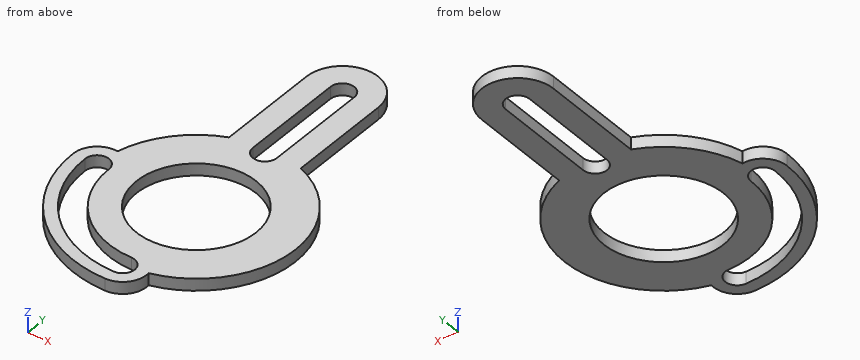
from build123d import *

# Parameters (mm, degrees)
SKETCH2_R           = 25
BOSS_EXTRUDE1_DEPTH = 5


with BuildPart() as part:
    # Sketch2 → Boss-Extrude1 (new body)
    with BuildSketch(Plane.XY):
        with BuildLine():
            Line((15, 82.39), (15, 38.694314828))
            ThreePointArc((15, 38.694314828), (41.414681799, -2.659723947), (9.927155207, -40.295180723))
            ThreePointArc((9.927155207, -40.295180723), (7.484924608, -48.131432999), (0, -51.5))
            ThreePointArc((0, -51.5), (-36.415999231, -36.415999231), (-51.5, 0))
            ThreePointArc((-51.5, 0), (-48.131432999, 7.484924608), (-40.295180723, 9.927155207))
            ThreePointArc((-40.295180723, 9.927155207), (-31.16531118, 27.403893502), (-15, 38.694314828))
            Line((-15, 38.694314828), (-15, 82.39))
            ThreePointArc((-15, 82.39), (0, 97.39), (15, 82.39))
        make_face()
        Circle(SKETCH2_R, mode=Mode.SUBTRACT)
        with BuildLine():
            Line((-5, 38.69), (-5, 82.39))
            ThreePointArc((-5, 82.39), (0, 87.39), (5, 82.39))
            Line((5, 82.39), (5, 38.69))
            ThreePointArc((5, 38.69), (0, 33.69), (-5, 38.69))
        make_face(mode=Mode.SUBTRACT)
        with BuildLine():
            ThreePointArc((-46.5, 0), (-32.880465325, -32.880465325), (0, -46.5))
            ThreePointArc((0, -46.5), (5, -41.5), (0, -36.5))
            ThreePointArc((0, -36.5), (-25.809397513, -25.809397513), (-36.5, 0))
            ThreePointArc((-36.5, 0), (-41.5, 5), (-46.5, 0))
        make_face(mode=Mode.SUBTRACT)
    extrude(amount=BOSS_EXTRUDE1_DEPTH)


solid = part.part
For this review, take the finished solid that the model builds, in its own axes (mm). Round coordinates to 2 decimals unless told otherwise and drop trailing zeros. Loops run counter-clockwise (first coordinate to the right, second up) from the corner with the lowest first, then second, coordinate; pieces in that order, holes last. Notation, with made-up numbers: (38, 26.5) - (69, 26.5) arc R27 ccw to (69, 56.5) - close; hole circle Ø4 at (23, -9). An arc over 180 degrees is marked (long way). Use one line per item in the form item = value.
Item 1: Consider section A-A on z = 0.95. Write out the cut boundary in (x, y).
Answers:
outline = (-51.5, 0) arc R51.5 ccw to (0, -51.5) arc R10 ccw to (9.93, -40.3) arc R41.5 ccw to (15, 38.69) - (15, 82.39) arc R15 ccw to (-15, 82.39) - (-15, 38.69) arc R41.5 ccw to (-40.3, 9.93) arc R10 ccw to start; hole (-46.5, 0) arc R46.5 ccw to (0, -46.5) arc R5 ccw to (0, -36.5) arc R36.5 cw to (-36.5, 0) arc R5 ccw to start; hole circle Ø50 at (0, 0); hole (-5, 38.69) arc R5 ccw to (5, 38.69) - (5, 82.39) arc R5 ccw to (-5, 82.39) - close
Item 2: Consider section D-D on x = -3. Write out the cut boundary in (y, z).
Answers:
outline = (-51.41, 0) - (-46.4, 0) - (-46.4, 5) - (-51.41, 5) - close; (-36.38, 0) - (-24.82, 0) - (-24.82, 5) - (-36.38, 5) - close; (24.82, 0) - (34.69, 0) - (34.69, 5) - (24.82, 5) - close; (86.39, 0) - (97.09, 0) - (97.09, 5) - (86.39, 5) - close
Item 3: Clearance check with flat-ended pins moving along their axes: P1, Ø1, axis at y = 14.5, z = 1.5, coming from the -X side; P2, Ø1, axis at y = 20.5, z = 3, coming from the -X side; P3, Ø1.5, axis at y = 69.5, z = 1.5, coming from the -X side; P4, Ø1.5, axis at x = 6, y = 22.5, coming from the +Z side. State where each tip first meets the part, or that it passes through.
Answers:
P1 = -39.07
P2 = -36.36
P3 = -15
P4 = through
Item 4: Consider section C-C on y = -15. Write out the cut boundary in (x, z), then the cut area to 3 significant figures.
Answers:
outline = (-49.27, 0) - (-44.01, 0) - (-44.01, 5) - (-49.27, 5) - close; (-33.28, 0) - (-20, 0) - (-20, 5) - (-33.28, 5) - close; (20, 0) - (38.69, 0) - (38.69, 5) - (20, 5) - close
area = 186 mm^2
Item 5: For line 1 (Y direction, x = -16, z = 2.65); line 2 (Y direction, x = -7.5, z = 1.25); line 3 (X direction, y = 85, z = 1.4), list the stretches that pass through material, from the lowest coordinate up.
Answers:
line_1 = -48.95 to -43.66, -32.81 to -19.21, 19.21 to 38.29
line_2 = -50.95 to -45.89, -35.72 to -23.85, 23.85 to 95.38
line_3 = -14.77 to -4.26, 4.26 to 14.77
Item 6: Consider section B-B on x = -18. Write out the cut boundary in (y, z), then the cut area to 3 significant figures.
Answers:
outline = (-48.25, 0) - (-42.87, 0) - (-42.87, 5) - (-48.25, 5) - close; (-31.75, 0) - (-17.35, 0) - (-17.35, 5) - (-31.75, 5) - close; (17.35, 0) - (37.39, 0) - (37.39, 5) - (17.35, 5) - close
area = 199 mm^2
